from build123d import *

# Parameters (mm, degrees)
SKETCH1_W           = 25.4
SKETCH1_H           = 88.9
SKETCH1_R           = 1.905
SKETCH1_W_2         = 19.558
SKETCH1_H_2         = 40.132
BOSS_EXTRUDE1_DEPTH = 19.177


with BuildPart() as part:
    # Sketch1 → Boss-Extrude1 (new body)
    with BuildSketch(Plane(origin=(0, 0, 0), x_dir=(1, 0, 0), z_dir=(0, 1, 0))):
        with Locations((12.7, 44.45)):
            Rectangle(SKETCH1_W, SKETCH1_H)
        with Locations(Location((6.731, 52.832, 0), (0, 0, 90))):
            Circle(SKETCH1_R, mode=Mode.SUBTRACT)
        with Locations(Location((18.669, 52.832, 0), (0, 0, 90))):
            Circle(SKETCH1_R, mode=Mode.SUBTRACT)
        with Locations(Location((6.731, 5.08, 0), (0, 0, 90))):
            Circle(SKETCH1_R, mode=Mode.SUBTRACT)
        with Locations(Location((18.669, 5.08, 0), (0, 0, 90))):
            Circle(SKETCH1_R, mode=Mode.SUBTRACT)
        with Locations((12.7, 28.956)):
            Rectangle(SKETCH1_W_2, SKETCH1_H_2, mode=Mode.SUBTRACT)
    extrude(amount=BOSS_EXTRUDE1_DEPTH)


solid = part.part
Verification items for the finished model (mm, model axes). A direction names the side the tool comes from. Coordinates: 2 decimals unless noted, no trailing zeros. Order: outer loops, then holes, each group sorted by start corner. A loop starts at its lowest first (then second) coordinate and runs counter-clockwise, first axis right, second up. Notation, with made-up numbers: (81.25, -36) -> (117.25, -36) arc R28 ccw to (117.25, -8) -> close; hole circle Ø9 at (-35, 21). An arc over 180 degrees is marked (long way). Use CSV: the item, a comma, the result in double quotes. Start each with the question number.
Q1. Draft check along Z on faces 1 (the cylindrical face through (6.647, 9.454, -3.177)), 2 (the flat face through (13, 9, -49.022)), 3 (the flat face through (13, 9, 0)), 4 (the flat face through (25.4, 9, -44)). Enter one of: +Z half, -Z half, draft (parallel to the pull), parting line (faces both ways), or undercut.
Q2. Section check C-C, the plane z = -14. Record the cut outline in (x, y), and give its area (3 significant figures).
Q3. Section check B-B, the plane z = -5.08. Record the cut outline in (x, y).
Q4. Thickness scan on line 1 along X through (y, z) = (11.5, -5.08); line 2 along Z through (x, y) = (6.5, 1.5); line 3 along Z through (x, y) = (15, 5.75). Record the ranges inside material, lowest first.
Q5. Section check D-D, the plane y = 16.5. Record the cut outline in (x, z) (3 decimals), and give its area (3 significant figures).
Q6. Tool access check on faces 5 (the flat face through (13, 9, -8.89)), 6 (the flat face through (13, 0, -55)). Record the directions out of +Z, -Z, +X, -X, +Y, -Y that give a thin tool (end or side, any length) a straight path to the whole face; none if there is none.
Q7. Section check A-A, the plane x = 13.75. Record the cut outline in (y, z), and give its area (3 significant figures).
Q8. Depth check by flat-ended pin: P1, Ø6, axis at y = 5.5, z = -64.5, coming from the -X side; P2, Ø2.5, axis at x = 18.669, z = -52.832, coming from the +Y side. Enter the tip coordinate at first touch or a pass-through.
Returned:
1,face 1,"undercut"
1,face 2,"undercut"
1,face 3,"+Z half"
1,face 4,"draft"
2,outline,"(0, 0) -> (2.92, 0) -> (2.92, 19.18) -> (0, 19.18) -> close; (22.48, 0) -> (25.4, 0) -> (25.4, 19.18) -> (22.48, 19.18) -> close"
2,area,"112 mm^2"
3,outline,"(0, 0) -> (4.83, 0) -> (4.83, 19.18) -> (0, 19.18) -> close; (8.64, 0) -> (16.76, 0) -> (16.76, 19.18) -> (8.64, 19.18) -> close; (20.57, 0) -> (25.4, 0) -> (25.4, 19.18) -> (20.57, 19.18) -> close"
4,line 1,"x = 0 to 4.83, 8.64 to 16.76, 20.57 to 25.4"
4,line 2,"z = -88.9 to -54.72, -50.94 to -49.02, -8.89 to -6.97, -3.19 to 0"
4,line 3,"z = -88.9 to -49.02, -8.89 to 0"
5,outline,"(0, -88.9) -> (25.4, -88.9) -> (25.4, 0) -> (0, 0) -> close; hole (2.921, -49.022) -> (22.479, -49.022) -> (22.479, -8.89) -> (2.921, -8.89) -> close; hole circle Ø3.81 at (6.731, -52.832); hole circle Ø3.81 at (6.731, -5.08); hole circle Ø3.81 at (18.669, -52.832); hole circle Ø3.81 at (18.669, -5.08)"
5,area,"1,430 mm^2"
6,face 5,"+Y, -Y"
6,face 6,"+Z, -Z, +X, -X, -Y"
7,outline,"(0, -88.9) -> (19.18, -88.9) -> (19.18, -49.02) -> (0, -49.02) -> close; (0, -8.89) -> (19.18, -8.89) -> (19.18, 0) -> (0, 0) -> close"
7,area,"935 mm^2"
8,P1,"stops at x = 0"
8,P2,"passes through"
